Here's the drawing with two shaded views (mm, measured from the low corner). I have some questions. Round coordinates to 2 decimals unless told otherwise and drop trailing zeros. Loops run counter-clockwise (first coordinate to the right, second up) from the corner with the lowest first, then second, coordinate; pieces in that order, holes last. Notation, with made-up numbers: (78, 49.25) -> (126, 49.25) arc R25 ccw to (126, 64.25) -> close; hole circle Ø11 at (-17.75, 58.5). An arc over 180 degrees is marked (long way). Use a Markdown table: item, result.
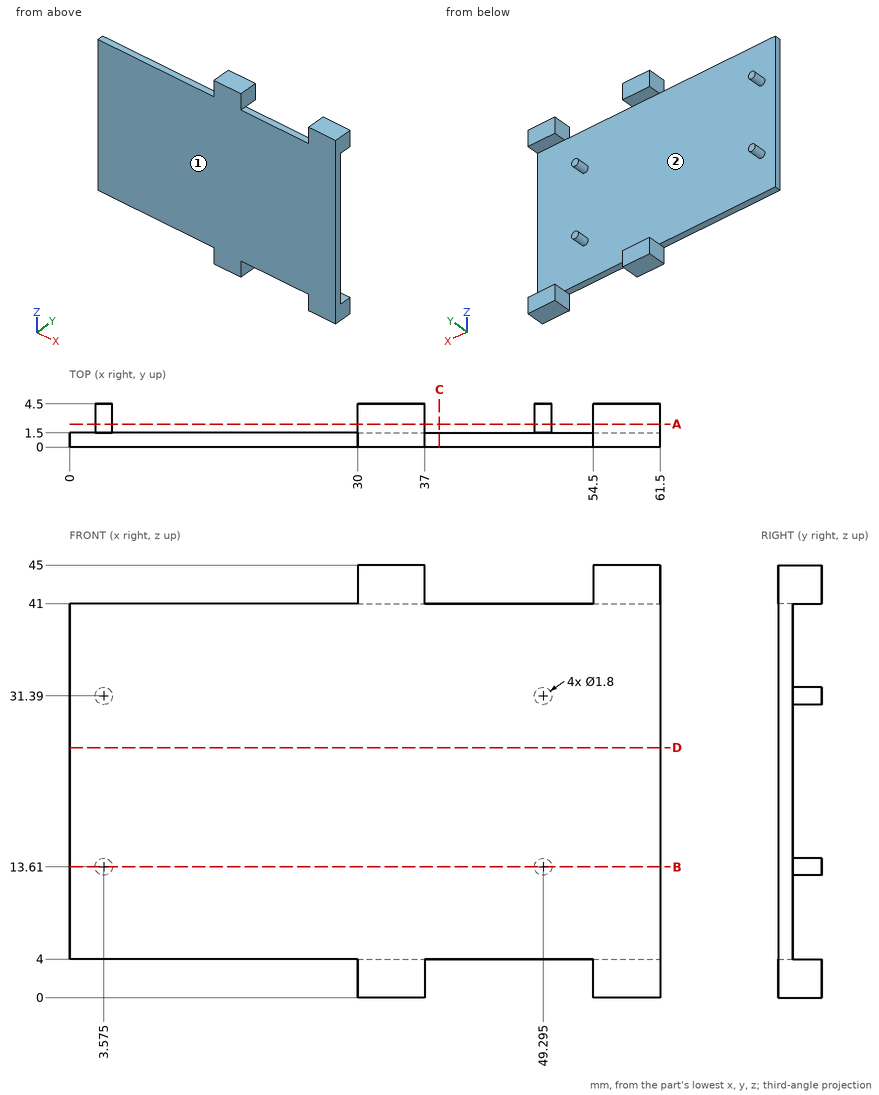
1. Will these pins go through, and if not, where does the flat tip stop? pin 1 Ø6 at (x, z) = (33, 17) entering from +Y; pin 2 Ø1.5 at (x, y) = (57.5, 3) entering from -Z; pin 3 Ø1.6 at (x, y) = (47, 1) entering from -Z; pin 4 Ø2 at (y, z) = (2.5, 1) entering from -X.
Answer sheet:
| item | result |
|---|---|
| pin 1 | stops at y = 1.5 |
| pin 2 | stops at z = 0 |
| pin 3 | stops at z = 4 |
| pin 4 | stops at x = 30 |
2. I want a section at B-B (z = 13.61). Please give me the cut outline in (x, y) (1 decimal).
Answer sheet:
| item | result |
|---|---|
| outline | (0, 0) -> (61.5, 0) -> (61.5, 1.5) -> (50.2, 1.5) -> (50.2, 4.5) -> (48.4, 4.5) -> (48.4, 1.5) -> (4.5, 1.5) -> (4.5, 4.5) -> (2.7, 4.5) -> (2.7, 1.5) -> (0, 1.5) -> close |
3. I want a section at C-C (x = 38.5). Please give me the cut outline in (y, z).
Answer sheet:
| item | result |
|---|---|
| outline | (0, 4) -> (1.5, 4) -> (1.5, 41) -> (0, 41) -> close |
4. I need wall thicknesses on line 1 (Z direction, x = 55, y = 3.3); line 2 (Z direction, x = 3.5, y = 3.2); line 3 (X direction, y = 0.7, z = 43). Which ranges of each line are inside material? Lowest first, please.
Answer sheet:
| item | result |
|---|---|
| line 1 | z = 0 to 4, 41 to 45 |
| line 2 | z = 12.71 to 14.51, 30.49 to 32.29 |
| line 3 | x = 30 to 37, 54.5 to 61.5 |
5. If we mould it in two halves opening along Z, with no side actions, what happens to the marked faces 1 and 2? For each: +Z half, -Z half, draft (parallel to the pull), parting line (faces both ways), or undercut.
Answer sheet:
| item | result |
|---|---|
| face 1 | draft |
| face 2 | undercut |
6. I want a section at A-A (y = 2.4). Please give me the cut outline in (x, z) (1 decimal), plus the area to 3 significant figures.
Answer sheet:
| item | result |
|---|---|
| outline | circle Ø1.8 at (3.6, 13.6); circle Ø1.8 at (3.6, 31.4); (30, 0) -> (37, 0) -> (37, 4) -> (30, 4) -> close; (30, 41) -> (37, 41) -> (37, 45) -> (30, 45) -> close; circle Ø1.8 at (49.3, 13.6); circle Ø1.8 at (49.3, 31.4); (54.5, 0) -> (61.5, 0) -> (61.5, 4) -> (54.5, 4) -> close; (54.5, 41) -> (61.5, 41) -> (61.5, 45) -> (54.5, 45) -> close |
| area | 122 mm² |
7. I want a section at D-D (z = 26). Please give me the cut outline in (x, y).
Answer sheet:
| item | result |
|---|---|
| outline | (0, 0) -> (61.5, 0) -> (61.5, 1.5) -> (0, 1.5) -> close |
